from build123d import *

# Parameters (mm, degrees)
ESQUISSE1_W               = 160
ESQUISSE1_H               = 160
BOSS_EXTRU_1_DEPTH        = 5
CHANFREIN3_SIZE           = 22
CHANFREIN4_SIZE           = 22
ENL_V_MAT_EXTRU_1_DEPTH   = 5
SYM_TRIE2_COPY_1_DEPTH    = 5
ESQUISSE8_R               = 2.5
ENL_V_MAT_EXTRU_2_DEPTH   = 5
SYM_TRIE4_COPY_1_SKETCH_R = 2.5
SYM_TRIE4_COPY_1_DEPTH    = 5
ESQUISSE9_R               = 2.5
ENL_V_MAT_EXTRU_3_DEPTH   = 5
SYM_TRIE6_COPY_1_SKETCH_R = 2.5
SYM_TRIE6_COPY_1_DEPTH    = 5
ESQUISSE10_R              = 2.5
ENL_V_MAT_EXTRU_4_DEPTH   = 10
ESQUISSE12_R              = 2.5
ENL_V_MAT_EXTRU_5_DEPTH   = 10


with BuildPart() as part:
    # Esquisse1 → Boss.-Extru.1 (new body)
    with BuildSketch(Plane.XY):
        with Locations((80, -80)):
            Rectangle(ESQUISSE1_W, ESQUISSE1_H)
    extrude(amount=BOSS_EXTRU_1_DEPTH)

    # Chanfrein3
    chanfrein3_edges = [part.edges().sort_by_distance(p)[0] for p in [
        (0, 0, 2.5),
    ]]
    chamfer(chanfrein3_edges, length=CHANFREIN3_SIZE)

    # Chanfrein4
    chanfrein4_edges = [part.edges().sort_by_distance(p)[0] for p in [
        (160, 0, 2.5),
        (160, -160, 2.5),
        (0, -160, 2.5),
    ]]
    chamfer(chanfrein4_edges, length=CHANFREIN4_SIZE)

    # Esquisse3 → Enlèv. mat.-Extru.1 (cut)
    with BuildSketch(Plane.XY.offset(5)):
        Polygon((25.143089642, -10.999045981), (11.000954019, -25.141181605), (39.285225266, -53.425452853), (53.42736089, -39.283317229), align=None)
    enl_v_mat_extru_1 = extrude(amount=-ENL_V_MAT_EXTRU_1_DEPTH, mode=Mode.SUBTRACT)

    # Symétrie1: Enlèv. mat.-Extru.1 across plane
    add(enl_v_mat_extru_1.mirror(Plane.ZX.offset(-80)), mode=Mode.SUBTRACT)

    # Symétrie2: Enlèv. mat.-Extru.1 across plane
    add(enl_v_mat_extru_1.mirror(Plane(origin=(80, 0, 0), x_dir=(0, 0, 1), z_dir=(1, 0, 0))), mode=Mode.SUBTRACT)

    # Symétrie2 copy 1 sketch → Symétrie2 copy 1 (cut)
    with BuildSketch(Plane(origin=(160, -160, 5), x_dir=(-1, 0, 0), z_dir=(0, 0, 1))):
        Polygon((25.143089642, -10.999045981), (11.000954019, -25.141181605), (39.285225266, -53.425452853), (53.42736089, -39.283317229), align=None)
    extrude(amount=-SYM_TRIE2_COPY_1_DEPTH, mode=Mode.SUBTRACT)

    # Esquisse8 → Enlèv. mat.-Extru.2 (cut)
    with BuildSketch(Plane.XY.offset(5)):
        with Locations((10.647400628, -18.423667184)):
            Circle(ESQUISSE8_R)
        with Locations((18.425575221, -10.645492591)):
            Circle(ESQUISSE8_R)
    enl_v_mat_extru_2 = extrude(amount=-ENL_V_MAT_EXTRU_2_DEPTH, mode=Mode.SUBTRACT)

    # Symétrie3: Enlèv. mat.-Extru.2 across plane
    add(enl_v_mat_extru_2.mirror(Plane.ZX.offset(-80)), mode=Mode.SUBTRACT)

    # Symétrie4: Enlèv. mat.-Extru.2 across plane
    add(enl_v_mat_extru_2.mirror(Plane(origin=(80, 0, 0), x_dir=(0, 0, 1), z_dir=(1, 0, 0))), mode=Mode.SUBTRACT)

    # Symétrie4 copy 1 sketch → Symétrie4 copy 1 (cut)
    with BuildSketch(Plane(origin=(160, -160, 5), x_dir=(-1, 0, 0), z_dir=(0, 0, 1))):
        with Locations((10.647400628, -18.423667184)):
            Circle(SYM_TRIE4_COPY_1_SKETCH_R)
        with Locations((18.425575221, -10.645492591)):
            Circle(SYM_TRIE4_COPY_1_SKETCH_R)
    extrude(amount=-SYM_TRIE4_COPY_1_DEPTH, mode=Mode.SUBTRACT)

    # Esquisse9 → Enlèv. mat.-Extru.3 (cut)
    with BuildSketch(Plane.XY.offset(5)):
        with Locations((53.78091428, -46.00083165)):
            Circle(ESQUISSE9_R)
        with Locations((46.002739687, -53.779006243)):
            Circle(ESQUISSE9_R)
    enl_v_mat_extru_3 = extrude(amount=-ENL_V_MAT_EXTRU_3_DEPTH, mode=Mode.SUBTRACT)

    # Symétrie5: Enlèv. mat.-Extru.3 across plane
    add(enl_v_mat_extru_3.mirror(Plane.ZX.offset(-80)), mode=Mode.SUBTRACT)

    # Symétrie6: Enlèv. mat.-Extru.3 across plane
    add(enl_v_mat_extru_3.mirror(Plane(origin=(80, 0, 0), x_dir=(0, 0, 1), z_dir=(1, 0, 0))), mode=Mode.SUBTRACT)

    # Symétrie6 copy 1 sketch → Symétrie6 copy 1 (cut)
    with BuildSketch(Plane(origin=(160, -160, 5), x_dir=(-1, 0, 0), z_dir=(0, 0, 1))):
        with Locations((53.78091428, -46.00083165)):
            Circle(SYM_TRIE6_COPY_1_SKETCH_R)
        with Locations((46.002739687, -53.779006243)):
            Circle(SYM_TRIE6_COPY_1_SKETCH_R)
    extrude(amount=-SYM_TRIE6_COPY_1_DEPTH, mode=Mode.SUBTRACT)

    # Esquisse10 → Enlèv. mat.-Extru.4 (cut)
    with BuildSketch(Plane.XY.offset(5)):
        with Locations((79.885822331, -34.038059223)):
            Circle(ESQUISSE10_R)
        with Locations((33.923881554, -80)):
            Circle(ESQUISSE10_R)
        with Locations((79.885822331, -125.961940777)):
            Circle(ESQUISSE10_R)
        with Locations((125.847763109, -80)):
            Circle(ESQUISSE10_R)
    extrude(amount=-ENL_V_MAT_EXTRU_4_DEPTH, mode=Mode.SUBTRACT)

    # Esquisse12 → Enlèv. mat.-Extru.5 (cut)
    with BuildSketch(Plane.XY.offset(5)):
        with Locations((5, -80)):
            Circle(ESQUISSE12_R)
        with Locations((155, -80)):
            Circle(ESQUISSE12_R)
        with Locations((80, -155)):
            Circle(ESQUISSE12_R)
        with Locations((80, -5)):
            Circle(ESQUISSE12_R)
    extrude(amount=-ENL_V_MAT_EXTRU_5_DEPTH, mode=Mode.SUBTRACT)


solid = part.part
Geometry: final body of the model. Coordinates: model frame, mm. A direction names the side the tool comes from. Round coordinates to 2 decimals unless told otherwise and drop trailing zeros. Order: outer loops, then holes, each group sorted by start corner. A loop starts at its lowest first (then second) coordinate and runs counter-clockwise, first axis right, second up. Notation, with made-up numbers: (17.25, 24) -> (51.25, 24) arc R31 ccw to (51.25, 54) -> close; hole circle Ø8 at (45.25, 61.5). An arc over 180 degrees is marked (long way). Put each result on its own line as item: value. Start each with the question number.
Q1. Pull-direction query (X, two-part tool) for faces 3 (the cylindrical face through (48.31, -54.74, 2.54)), 4 (the flat face through (79, -79, 0)), 5 (the flat face through (149, -149, 2)); classes: +X half, -X half, draft (parallel to the pull), parting line (faces both ways), or undercut.
Q2. Section C-C on y = -80. Return the cut outline in (x, z), and give its area (3 significant figures).
Q3. First-contact query: pin 1 (8 mm diameter, centred on x = 5, y = -80, fed in from -Z). Flat tip, straight axial feed; report the tip coordinate or a pass-through.
Q4. Section B-B on x = 5. Return the cut outline in (y, z), and give its area (3 significant figures).
Q5. Line query: probe 1 along Y at (x, z) = (80, 1.5); probe 2 along Y at (x, z) = (78.5, 4.7); probe 3 along X at (y, z) = (-133.5, 3.2). Output: solid intervals per line, ascending.
Q6. Section A-A on y = -155. Return the cut outline in (x, z), and give its area (3 significant figures).
Q7. Section D-D on x = 27.5. Return the cut outline in (y, z), and give its area (3 significant figures).
Q8. Reachability of faces 1 (the flat face through (11, -149, 2)), 2 (the flat face through (39.483, -25.339, 2.535)) from +Z, -Z, +X, -X, +Y, -Y: full face, straight path, thin tool, end or side. Return the list, or none.
Ans:
1. face 3: undercut
1. face 4: draft
1. face 5: +X half
2. outline: (0, 0) -> (2.5, 0) -> (2.5, 5) -> (0, 5) -> close; (7.5, 0) -> (31.42, 0) -> (31.42, 5) -> (7.5, 5) -> close; (36.42, 0) -> (123.35, 0) -> (123.35, 5) -> (36.42, 5) -> close; (128.35, 0) -> (152.5, 0) -> (152.5, 5) -> (128.35, 5) -> close; (157.5, 0) -> (160, 0) -> (160, 5) -> (157.5, 5) -> close
2. area: 700 mm2
3. pin 1: stops at z = 0
4. outline: (-143, 0) -> (-82.5, 0) -> (-82.5, 5) -> (-143, 5) -> close; (-77.5, 0) -> (-17, 0) -> (-17, 5) -> (-77.5, 5) -> close
4. area: 605 mm2
5. probe 1: y = -160 to -157.5, -152.5 to -128.46, -123.46 to -36.54, -31.54 to -7.5, -2.5 to 0
5. probe 2: y = -160 to -157, -153 to -128.04, -123.88 to -36.12, -31.96 to -7, -3 to 0
5. probe 3: x = 0 to 12.36, 40.64 to 119.36, 147.64 to 160
6. outline: (17, 0) -> (77.5, 0) -> (77.5, 5) -> (17, 5) -> close; (82.5, 0) -> (143, 0) -> (143, 5) -> (82.5, 5) -> close
6. area: 605 mm2
7. outline: (-160, 0) -> (-146.64, 0) -> (-146.64, 5) -> (-160, 5) -> close; (-118.36, 0) -> (-41.64, 0) -> (-41.64, 5) -> (-118.36, 5) -> close; (-13.36, 0) -> (0, 0) -> (0, 5) -> (-13.36, 5) -> close
7. area: 517 mm2
8. face 1: +Z, -Z, -X, -Y
8. face 2: +Z, -Z
